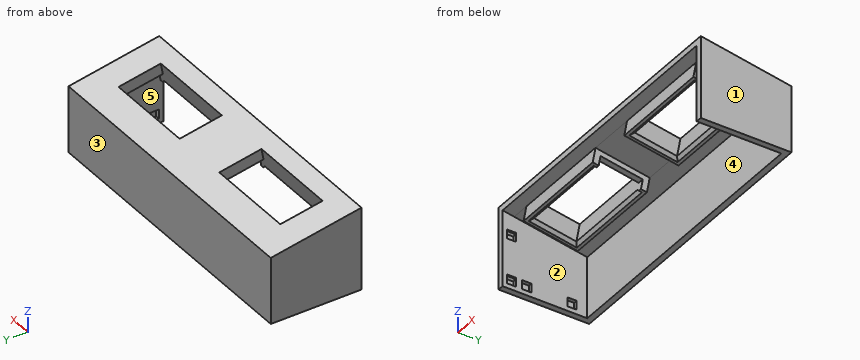
```python
from build123d import *

# Parameters (mm, degrees)
SKETCH1_W               = 100
SKETCH1_H               = 45
BOSS_EXTRUDE1_DEPTH     = 30
CUT_EXTRUDE5_DEPTH      = 107.800046816
SKETCH2_W               = 30.2
SKETCH2_H               = 14.2
CUT_EXTRUDE1_DEPTH      = 61.848905169
CUT_EXTRUDE6_REACH      = 64.5
SKETCH9_W               = 96
SKETCH9_H               = 41
SHELL2_START            = -48
SHELL2_DEPTH            = 96
SHELL2_START_2          = -7.8
SHELL2_2_DEPTH          = 15.6
SHELL2_3_DEPTH          = 6
SHELL2_START_3          = 42
SHELL2_4_DEPTH          = 6
SKETCH10_W              = 96
SKETCH10_H              = 2
CUT_EXTRUDE7_DEPTH      = 2
CUT_EXTRUDE9_START      = -1.5
SKETCH12_W              = 1.25
SKETCH12_H              = 3
CUT_EXTRUDE9_DEPTH      = 3
LPATTERN2_COUNT         = 2
LPATTERN2_PITCH         = 15
LPATTERN3_COUNT         = 2
LPATTERN3_PITCH         = 5
LPATTERN4_COUNT         = 2
LPATTERN4_PITCH         = 20
MIRROR7_START           = -1.5
MIRROR7_COPY_1_SKETCH_W = 1.25
MIRROR7_COPY_1_SKETCH_H = 3
MIRROR7_COPY_1_DEPTH    = 3
MIRROR7_COPY_2_SKETCH_W = 1.25
MIRROR7_COPY_2_SKETCH_H = 3
MIRROR7_COPY_2_DEPTH    = 3
MIRROR7_COPY_3_SKETCH_W = 1.25
MIRROR7_COPY_3_SKETCH_H = 3
MIRROR7_COPY_3_DEPTH    = 3
CHAMFER4_SIZE           = 1
SKETCH13_W              = 30
SKETCH13_H              = 15
CUT_EXTRUDE10_DEPTH     = 107.800046816
CHAMFER5_SIZE           = 0.6
SKETCH14_W              = 2
SKETCH14_H              = 14.2
CUT_EXTRUDE11_DEPTH     = 3.5


# Read off the part's stored shape, not the designer's step: Shell2
with BuildPart() as part:
    # Sketch1 → Boss-Extrude1 (new body)
    with BuildSketch(Plane.XY):
        Rectangle(SKETCH1_W, SKETCH1_H)
    extrude(amount=BOSS_EXTRUDE1_DEPTH)

    # Sketch7 → Cut-Extrude5 (cut, through all)
    with BuildSketch(Plane(origin=(50, 0, 0), x_dir=(0, 0, -1), z_dir=(1, 0, 0))):
        Polygon((-30, -22.5), (-22.065285868, 22.5), (-30, 22.5), align=None)
    extrude(amount=-CUT_EXTRUDE5_DEPTH, mode=Mode.SUBTRACT)

    # Sketch2 → Cut-Extrude1 (cut, through all)
    with BuildSketch(Plane(origin=(0, -0.341825557, 26.092916002), x_dir=(1, 0, 0), z_dir=(0, 0.17364817766692325, 0.9848077530122092))):
        with Locations((-24.9, 6.094197535)):
            Rectangle(SKETCH2_W, SKETCH2_H)
    cut_extrude1 = extrude(amount=-CUT_EXTRUDE1_DEPTH, mode=Mode.SUBTRACT)

    # Mirror1: Cut-Extrude1 across plane
    add(cut_extrude1.mirror(Plane(origin=(0, 0, 0), x_dir=(0, 0, 1), z_dir=(1, 0, 0))), mode=Mode.SUBTRACT)

    # Cut-Extrude6: up to this plane
    cut_extrude6_end = Plane(origin=(-50, -23.767631697, 22.810903403), z_dir=(0, -0.17364817766692328, -0.9848077530122092))
    # Sketch9 → Cut-Extrude6 (cut, up to the surface)
    with BuildSketch(Plane(origin=(0, 0, 0), x_dir=(-1, 0, 0), z_dir=(0, 0, -1)), mode=Mode.PRIVATE) as cut_extrude6_sk1:
        Rectangle(SKETCH9_W, SKETCH9_H)
    cut_extrude6_tool1 = split(extrude(cut_extrude6_sk1.sketch, amount=-CUT_EXTRUDE6_REACH, mode=Mode.PRIVATE), bisect_by=cut_extrude6_end, keep=Keep.BOTH, mode=Mode.PRIVATE)
    add(cut_extrude6_tool1.solids().sort_by_distance((0, 0, 0))[0], mode=Mode.SUBTRACT)

    # Shell2 outline → Shell2 (cut)
    with BuildSketch(Plane.YZ.offset(SHELL2_START)):
        Polygon((13.353906279, 16.265374693), (20.5, 15.005325563), (20.5, 20.387086606), (14.274241621, 21.484855784), align=None)
        Polygon((-20.5, 22.234731772), (-4.569594826, 19.425771526), (-3.649259484, 24.645252617), (-22.5, 27.969146776), (-22.5, 2), (-20.5, 2), align=None)
    extrude(amount=SHELL2_DEPTH, mode=Mode.SUBTRACT)

    # Shell2 2 outline → Shell2 2 (cut)
    with BuildSketch(Plane.YZ.offset(SHELL2_START_2)):
        Polygon((-4.569594826, 19.425771526), (13.353906279, 16.265374693), (14.274241621, 21.484855783), (-3.649259484, 24.645252617), align=None)
    extrude(amount=SHELL2_2_DEPTH, mode=Mode.SUBTRACT)

    # Shell2 3 outline → Shell2 3 (cut)
    with BuildSketch(Plane.YZ.offset(SHELL2_START)):
        Polygon((-4.569594826, 19.425771526), (13.353906279, 16.265374693), (14.274241621, 21.484855783), (-3.649259484, 24.645252617), align=None)
    extrude(amount=SHELL2_3_DEPTH, mode=Mode.SUBTRACT)

    # Shell2 4 outline → Shell2 4 (cut)
    with BuildSketch(Plane.YZ.offset(SHELL2_START_3)):
        Polygon((-4.569594826, 19.425771526), (13.353906279, 16.265374693), (14.274241621, 21.484855783), (-3.649259484, 24.645252617), align=None)
    extrude(amount=SHELL2_4_DEPTH, mode=Mode.SUBTRACT)

    # Sketch10 → Cut-Extrude7 (cut)
    with BuildSketch(Plane(origin=(0, 0, 0), x_dir=(-1, 0, 0), z_dir=(0, 0, -1))):
        with Locations((0, -21.5)):
            Rectangle(SKETCH10_W, SKETCH10_H)
    extrude(amount=-CUT_EXTRUDE7_DEPTH, mode=Mode.SUBTRACT)

    # Sketch12 → Cut-Extrude9 (cut)
    with BuildSketch(Plane(origin=(0, 0, 0), x_dir=(-1, 0, 0), z_dir=(0, 0, -1)).offset(CUT_EXTRUDE9_START)):
        with Locations((48.625, -4.5)):
            Rectangle(SKETCH12_W, SKETCH12_H)
    cut_extrude9 = extrude(amount=-CUT_EXTRUDE9_DEPTH, mode=Mode.SUBTRACT)

    # LPattern2: Cut-Extrude9 ×2
    with Locations(*[(0, 0, i * LPATTERN2_PITCH) for i in range(1, LPATTERN2_COUNT)]):
        add(cut_extrude9, mode=Mode.SUBTRACT)

    # LPattern3: Cut-Extrude9 ×2
    with Locations(*[(0, i * LPATTERN3_PITCH, 0) for i in range(1, LPATTERN3_COUNT)]):
        add(cut_extrude9, mode=Mode.SUBTRACT)

    # LPattern4: Cut-Extrude9 ×2
    with Locations(*[(0, i * LPATTERN4_PITCH, 0) for i in range(1, LPATTERN4_COUNT)]):
        add(cut_extrude9, mode=Mode.SUBTRACT)

    # Mirror7: Cut-Extrude9 across plane
    add(cut_extrude9.mirror(Plane(origin=(0, 0, 0), x_dir=(0, 0, 1), z_dir=(1, 0, 0))), mode=Mode.SUBTRACT)

    # Mirror7 copy 1 sketch → Mirror7 copy 1 (cut)
    with BuildSketch(Plane(origin=(0, 0, 15), x_dir=(1, 0, 0), z_dir=(0, 0, -1)).offset(MIRROR7_START)):
        with Locations((48.625, 4.5)):
            Rectangle(MIRROR7_COPY_1_SKETCH_W, MIRROR7_COPY_1_SKETCH_H)
    extrude(amount=-MIRROR7_COPY_1_DEPTH, mode=Mode.SUBTRACT)

    # Mirror7 copy 2 sketch → Mirror7 copy 2 (cut)
    with BuildSketch(Plane(origin=(0, 5, 0), x_dir=(1, 0, 0), z_dir=(0, 0, -1)).offset(MIRROR7_START)):
        with Locations((48.625, 4.5)):
            Rectangle(MIRROR7_COPY_2_SKETCH_W, MIRROR7_COPY_2_SKETCH_H)
    extrude(amount=-MIRROR7_COPY_2_DEPTH, mode=Mode.SUBTRACT)

    # Mirror7 copy 3 sketch → Mirror7 copy 3 (cut)
    with BuildSketch(Plane(origin=(0, 20, 0), x_dir=(1, 0, 0), z_dir=(0, 0, -1)).offset(MIRROR7_START)):
        with Locations((48.625, 4.5)):
            Rectangle(MIRROR7_COPY_3_SKETCH_W, MIRROR7_COPY_3_SKETCH_H)
    extrude(amount=-MIRROR7_COPY_3_DEPTH, mode=Mode.SUBTRACT)

    # Chamfer4
    chamfer4_edges = [part.edges().sort_by_distance(p)[0] for p in [
        (24.9, -2.59997932, 19.078475171),
        (9.8, 4.392155727, 17.845573109),
        (24.9, 11.384290773, 16.612671048),
        (40, 4.392155727, 17.845573109),
        (-24.9, -2.59997932, 19.078475171),
        (-9.8, 4.392155727, 17.845573109),
        (-24.9, 11.384290773, 16.612671048),
        (-40, 4.392155727, 17.845573109),
    ]]
    chamfer(chamfer4_edges, length=CHAMFER4_SIZE)

    # Sketch13 → Cut-Extrude10 (cut, through all)
    with BuildSketch(Plane.ZY.offset(50)):
        with Locations((15, -15)):
            Rectangle(SKETCH13_W, SKETCH13_H)
    extrude(amount=-CUT_EXTRUDE10_DEPTH, mode=Mode.SUBTRACT)

    # Chamfer5
    chamfer5_edges = [part.edges().sort_by_distance(p)[0] for p in [
        (-49.25, -4.5, 4.5),
        (-49.25, -4.5, 19.5),
        (49.25, -4.5, 4.5),
        (49.25, -4.5, 19.5),
    ]]
    chamfer(chamfer5_edges, length=CHAMFER5_SIZE)

    # Sketch14 → Cut-Extrude11 (cut)
    with BuildSketch(Plane(origin=(0, 3.184212437, 18.058566102), x_dir=(-1, 0, 0), z_dir=(0, -0.17364817766692328, -0.9848077530122094))):
        with Locations((8.8, 1.226577762)):
            Rectangle(SKETCH14_W, SKETCH14_H)
        with Locations((-41, 1.226577762)):
            Rectangle(SKETCH14_W, SKETCH14_H)
    extrude(amount=-CUT_EXTRUDE11_DEPTH, mode=Mode.SUBTRACT)


solid = part.part
```
For this review, take the finished solid that the model builds, in its own axes (mm). Face numbers are marked on the shaded views. A direction names the side the tool comes from. Give positions to 0.01 mm unless a question says otherwise; leave off trailing zeros. Write each loop counter-clockwise with the first axis right and the second up, starting at its lowest first coordinate (ties: lowest second). Pieces come first, ordered by that corner, then holes.
Item 1: Take a section at A-A (x = 30). Give the boundary of the cut face in (y, z), and give its area (3 significant figures).
Item 2: Take a section at C-C (x = -43). Give the boundary of the cut face in (y, z), and give its area (3 significant figures).
Item 3: Wall thickness on probe 1 along X at (y, z) = (-4.5, 22.5); probe 2 along X at (y, z) = (4, 20.5); probe 3 along Y at (x, z) = (-4.5, 4.75): over which ranges is each line inside the solid? List them lowest first.
Item 4: Take a section at D-D (z = 13). Give the boundary of the cut face in (x, y), and give its area (3 significant figures).
Item 5: Take a section at B-B (y = 0.5). Give the number of separate pieces and of enclosed holes in the cut face, and give its area (3 significant figures).
Item 6: Insertion check: P1, Ø8, axis at x = -15.5, y = -0.5, coming from the -Z side; P2, Ø1, axis at x = 33.5, z = 19, coming from the -Y side; P3, Ø1.5, axis at x = 0, z = 6.5, coming from the -Y side. Each pin has a flat end and moves straight along its axis. Give the tip position at first contact, or say it passes through.
Item 7: Machinability: for the marked faces 1 and 2, which of the approach directions +Z, -Z, +X, -X, +Y, -Y give a long, thin tool a straight path to every point of the face, cutting with its end or side? Answer none if there is none.
Item 8: The part is to be moulded in two halves that separate along Y. For the marked faces 3, 4 and 5, say which applies: +Y half, -Y half, draft (parallel to the pull), parting line (faces both ways), or undercut.
Established:
1. outline: (-7.5, 25.32) - (-3.65, 24.65) - (-4.57, 19.43) - (-3.58, 19.25) - (-2.43, 20.06) - (-1.33, 26.27) - (-7.5, 27.36) - close; (11.56, 17.6) - (12.37, 16.44) - (13.35, 16.27) - (14.27, 21.48) - (20.5, 20.39) - (20.5, 0) - (22.5, 0) - (22.5, 22.07) - (12.65, 23.8) - close
1. area: 93.1 mm2
2. outline: (-7.5, 25.32) - (20.5, 20.39) - (20.5, 0) - (22.5, 0) - (22.5, 22.07) - (-7.5, 27.36) - close
2. area: 101 mm2
3. probe 1: x = -50 to -48, 48 to 50
3. probe 2: x = -50 to -48, -42 to -40, 7.8 to 9.8, 48 to 50
3. probe 3: y = 20.5 to 22.5
4. outline: (-50, -7.5) - (-48, -7.5) - (-48, 20.5) - (48, 20.5) - (48, -7.5) - (50, -7.5) - (50, 22.5) - (-50, 22.5) - close
4. area: 312 mm2
5. separate pieces: 3
5. enclosed holes: 0
5. area: 196 mm2
6. P1: stops at z = 19.25
6. P2: stops at y = -4.57
6. P3: stops at y = 20.5
7. face 1: +Z, -Z, +X, +Y, -Y
7. face 2: -Z, -Y
8. face 3: +Y half
8. face 4: undercut
8. face 5: draft
